Source: CAD feature listing. Evaluate the final solid. Frame: model axes, mm. Face numbers are marked on the shaded views. A direction names the side the tool comes from. Coordinates: 2 decimals unless noted, no trailing zeros. Loops run counter-clockwise (first coordinate to the right, second up) from the corner with the lowest first, then second, coordinate; pieces in that order, holes last. Notation, with made-up numbers: (-40, -12) - (-33, -12) arc R31 cw to (-33, 27) - close; hole circle Ø11 at (71.5, 71.5). An arc over 180 degrees is marked (long way). Use one line per item in the form item = value. Start each with the question number.
from build123d import *

# Parameters (mm, degrees)
CROQUIS1_W     = 120
CROQUIS1_H     = 40
EXTRUIR1_DEPTH = 20
CROQUIS2_R     = 5
EXTRUIR2_DEPTH = 67.332495807
CROQUIS4_R     = 7.5
CROQUIS4_R_2   = 2.5
EXTRUIR3_DEPTH = 10


with BuildPart() as part:
    # Croquis1 → Extruir1 (new body)
    with BuildSketch(Plane(origin=(0, 0, 0), x_dir=(1, 0, 0), z_dir=(0, 1, 0))):
        Rectangle(CROQUIS1_W, CROQUIS1_H)
    extrude(amount=EXTRUIR1_DEPTH)

    # Croquis2 → Extruir2 (cut, through all)
    with BuildSketch(Plane(origin=(0, 20, 0), x_dir=(1, 0, 0), z_dir=(0, 1, 0))):
        with Locations(Location((-50, 0, 0), (0, 0, 270))):
            Circle(CROQUIS2_R)
        with Locations(Location((50, 0, 0), (0, 0, 90))):
            Circle(CROQUIS2_R)
    extrude(amount=-EXTRUIR2_DEPTH, mode=Mode.SUBTRACT)

    # Croquis4 → Extruir3 (cut)
    with BuildSketch(Plane(origin=(0, 20, 0), x_dir=(1, 0, 0), z_dir=(0, 1, 0))):
        with Locations(Location((-30, 0, 0), (0, 0, 270))):
            Circle(CROQUIS4_R)
        with Locations(Location((30, 0, 0), (0, 0, 90))):
            Circle(CROQUIS4_R)
        with Locations(Location((0, 0, 0), (0, 0, 270))):
            Circle(CROQUIS4_R_2)
    extrude(amount=-EXTRUIR3_DEPTH, mode=Mode.SUBTRACT)


solid = part.part
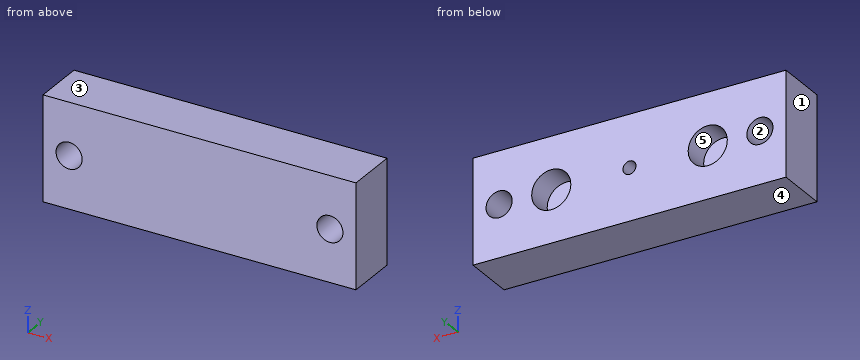
(1) Access query for the marked faces 4 and 5. Directions: +Z, -Z, +X, -X, +Y, -Y. A direction counts if a zero-diameter tool reaches every point of the face in a straight line with its end or side. Return the directions, or none.
(2) Material intervals for line 1 (X direction, y = 7, z = 0); line 2 (X direction, y = 18.25, z = 0); line 3 (Z direction, x = 30, y = 18), sorted ascending.
(3) Cut plane B-B, the plane y = 17.25. Output: boundary loops of the cut face in (x, z).
(4) Cut plane D-D, the plane x = -50. Output: boundary loops of the cut face in (y, z), plus the area to 3 significant figures.
(5) Cut plane A-A, the plane z = 0. Output: boundary loops of the cut face in (x, y), plus the area to 3 significant figures.
(6) Cut plane C-C, the plane x = 0. Output: boundary loops of the cut face in (y, z), plus the area to 3 significant figures.
(7) Mould query, pull axis X, two halves, no side actions, for the marked faces 1, 2 and 3. Classes: +X half, -X half, draft (parallel to the pull), parting line (faces both ways), or undercut.
(8) Contact query for flat-ended pins moving along their axis: pin 1 (9 mm diameter, centred on x = -30, z = 0, fed in from -Y); pin 2 (7.5 mm diameter, centred on x = 27, z = 1, fed in from +Y); pin 3 (8 mm diameter, centred on x = -50, z = 0, fed in from -Y). Output: stop coordinate, or through.
Recorded:
q1.face_4 = -Z, +X, -X, +Y, -Y
q1.face_5 = +Y
q2.line_1 = -60 to -55, -45 to 45, 55 to 60
q2.line_2 = -60 to -55, -45 to -37.5, -22.5 to -2.5, 2.5 to 22.5, 37.5 to 45, 55 to 60
q2.line_3 = -20 to -7.5, 7.5 to 20
q3.outline = (-60, -20) - (60, -20) - (60, 20) - (-60, 20) - close; hole circle Ø10 at (-50, 0); hole circle Ø15 at (-30, 0); hole circle Ø5 at (0, 0); hole circle Ø15 at (30, 0); hole circle Ø10 at (50, 0)
q4.outline = (0, -20) - (20, -20) - (20, -5) - (0, -5) - close; (0, 5) - (20, 5) - (20, 20) - (0, 20) - close
q4.area = 600 mm²
q5.outline = (-60, 0) - (-55, 0) - (-55, 20) - (-60, 20) - close; (-45, 0) - (45, 0) - (45, 20) - (37.5, 20) - (37.5, 10) - (22.5, 10) - (22.5, 20) - (2.5, 20) - (2.5, 10) - (-2.5, 10) - (-2.5, 20) - (-22.5, 20) - (-22.5, 10) - (-37.5, 10) - (-37.5, 20) - (-45, 20) - close; (55, 0) - (60, 0) - (60, 20) - (55, 20) - close
q5.area = 1,650 mm²
q6.outline = (0, -20) - (20, -20) - (20, -2.5) - (10, -2.5) - (10, 2.5) - (20, 2.5) - (20, 20) - (0, 20) - close
q6.area = 750 mm²
q7.face_1 = -X half
q7.face_2 = undercut
q7.face_3 = draft
q8.pin_1 = 0
q8.pin_2 = 10
q8.pin_3 = through
